```python
from build123d import *

# Parameters (mm, degrees)
SKETCH1_W           = 24
SKETCH1_H           = 34
SKETCH1_R           = 7.5
BOSS_EXTRUDE1_DEPTH = 28
SKETCH3_W           = 30
SKETCH3_H           = 12
BOSS_EXTRUDE2_DEPTH = 35.15
SKETCH4_R           = 11
CUT_EXTRUDE2_DEPTH  = 8
FILLET1_R           = 2
SKETCH5_W           = 12
SKETCH5_H           = 30
BOSS_EXTRUDE3_DEPTH = 10
SKETCH6_W           = 8
SKETCH6_H           = 5
CUT_EXTRUDE3_DEPTH  = 74.076141797
CUT_EXTRUDE4_REACH  = 87.286
SKETCH7_R           = 1
SKETCH8_R           = 4
CUT_EXTRUDE5_DEPTH  = 20
SKETCH9_R           = 7
CUT_EXTRUDE6_DEPTH  = 10


with BuildPart() as part:
    # Sketch1 → Boss-Extrude1 (new, symmetric)
    with BuildSketch(Plane.XY):
        with Locations((0, -5)):
            Rectangle(SKETCH1_W, SKETCH1_H)
        Circle(SKETCH1_R, mode=Mode.SUBTRACT)
    extrude(amount=BOSS_EXTRUDE1_DEPTH, both=True)

    # Sketch3 → Boss-Extrude2 (add)
    with BuildSketch(Plane.XZ.offset(22)):
        with Locations((0, 7.5)):
            Rectangle(SKETCH3_W, SKETCH3_H)
    extrude(amount=BOSS_EXTRUDE2_DEPTH)

    # Sketch4 → Cut-Extrude2 (cut)
    with BuildSketch(Plane.XY.offset(13.5)):
        with Locations((0, -43.15)):
            Circle(SKETCH4_R)
    extrude(amount=-CUT_EXTRUDE2_DEPTH, mode=Mode.SUBTRACT)

    # Fillet1
    fillet1_edges = [part.edges().sort_by_distance(p)[0] for p in [
        (0, -22, 1.5),
        (0, -22, 13.5),
    ]]
    fillet(fillet1_edges, radius=FILLET1_R)

    # Sketch5 → Boss-Extrude3 (add)
    with BuildSketch(Plane(origin=(0, 12, 0), x_dir=(1, 0, 0), z_dir=(0, 1, 0))):
        with Locations((6, 0)):
            Rectangle(SKETCH5_W, SKETCH5_H)
    extrude(amount=BOSS_EXTRUDE3_DEPTH)

    # Sketch6 → Cut-Extrude3 (cut, through all)
    with BuildSketch(Plane.XY.offset(15)):
        with Locations((4, 14.5)):
            Rectangle(SKETCH6_W, SKETCH6_H)
    extrude(amount=-CUT_EXTRUDE3_DEPTH, mode=Mode.SUBTRACT)

    # Sketch7 → Cut-Extrude4 (cut, up to next)
    with BuildSketch(Plane(origin=(0, 22, 0), x_dir=(1, 0, 0), z_dir=(0, 1, 0)), mode=Mode.PRIVATE) as cut_extrude4_sk1:
        with Locations(Location((4, 11, 0), (0, 0, 270))):
            Circle(SKETCH7_R)
    cut_extrude4_tool1 = extrude(cut_extrude4_sk1.sketch, amount=-CUT_EXTRUDE4_REACH, mode=Mode.PRIVATE) & part.part
    # Sketch7 → Cut-Extrude4 (cut, up to next)
    with BuildSketch(Plane(origin=(0, 22, 0), x_dir=(1, 0, 0), z_dir=(0, 1, 0)), mode=Mode.PRIVATE) as cut_extrude4_sk2:
        with Locations(Location((4, -11, 0), (0, 0, 270))):
            Circle(SKETCH7_R)
    cut_extrude4_tool2 = extrude(cut_extrude4_sk2.sketch, amount=-CUT_EXTRUDE4_REACH, mode=Mode.PRIVATE) & part.part
    add(cut_extrude4_tool1.solids().sort_by_distance((4, 22, -11))[0], mode=Mode.SUBTRACT)
    add(cut_extrude4_tool2.solids().sort_by_distance((4, 22, 11))[0], mode=Mode.SUBTRACT)

    # Sketch8 → Cut-Extrude5 (cut)
    with BuildSketch(Plane(origin=(12, 0, 0), x_dir=(0, 0, -1), z_dir=(1, 0, 0))):
        with Locations(Location((-14, -14, 0), (0, 0, 90))):
            Circle(SKETCH8_R)
        with Locations(Location((14, -14, 0), (0, 0, 90))):
            Circle(SKETCH8_R)
    extrude(amount=-CUT_EXTRUDE5_DEPTH, mode=Mode.SUBTRACT)

    # Sketch9 → Cut-Extrude6 (cut)
    with BuildSketch(Plane.XY.offset(5.5)):
        with Locations((0, -43.15)):
            Circle(SKETCH9_R)
    extrude(amount=-CUT_EXTRUDE6_DEPTH, mode=Mode.SUBTRACT)


solid = part.part
```
Geometry check sheet. Reference: the model listing, model coordinates, mm. A direction names the side the tool comes from. Coordinates: 2 decimals unless noted, no trailing zeros. Order: outer loops, then holes, each group sorted by start corner. A loop starts at its lowest first (then second) coordinate and runs counter-clockwise, first axis right, second up.
Item 1: Section check D-D (y = -40.5). Enter the section's corners in (x, z), plus the area to 3 significant figures.
Item 2: Section check B-B (z = -14). Enter the section's corners in (x, y), plus the area to 3 significant figures.
Item 3: Section check C-C (z = 11). Enter the section's corners in (x, y).
Item 4: Scan lines: line 1 along Z through (x, y) = (0.25, -14); line 2 along Y through (x, z) = (-4.75, -12); line 3 along X through (y, z) = (20.55, -11). Record each from-to range of solid material in increasing order.
Item 5: Depth check by flat-ended pin: pin 1 (8 mm diameter, centred on y = 13, z = -13, fed in from -X); pin 2 (23 mm diameter, centred on y = 7.5, z = -4, fed in from +X); pin 3 (1.5 mm diameter, centred on x = -6, z = 10.5, fed in from +Y); pin 4 (2.5 mm diameter, centred on x = 4, z = 11, fed in from +Y). Enter the tip coordinate at first touch or a pass-through.
Item 6: Tool access check on faces 4 (the flat face through (8, 14, 0)), 5 (the cylindrical face through (5.076, -52.909, 9.556)), 6 (the flat face through (0, -22, 22)), 7 (the flat face through (-8, -14, -14)). Record the directions out of +Z, -Z, +X, -X, +Y, -Y that give a thin tool (end or side, any length) a straight path to the whole face; none if there is none.
Item 7: Mould release check, pull along Y, two halves, no side actions. Record for faces 1 (the flat face through (-0.2, -50.3, 5.5)), 2 (the flat face through (-14, -22, 8)), 3 (the cylindrical face through (4.676, 19.535, -11.737)): released by +Y, released by -Y, zero draft, split by the parting line, or undercut.
Item 8: Section check A-A (y = 0). Enter the section's corners in (x, z).
Check sheet entries:
1. outline: (-15, 1.5) - (-6.48, 1.5) - (-6.48, 5.5) - (-10.68, 5.5) - (-10.68, 13.5) - (-15, 13.5) - close; (6.48, 1.5) - (15, 1.5) - (15, 13.5) - (10.68, 13.5) - (10.68, 5.5) - (6.48, 5.5) - close
1. area: 137 mm2
2. outline: (-12, -22) - (12, -22) - (12, -18) - (-8, -18) - (-8, -10) - (12, -10) - (12, 22) - (0, 22) - (0, 17) - (8, 17) - (8, 12) - (-12, 12) - close; hole circle Ø15 at (0, 0)
2. area: 559 mm2
3. outline: (-15, -57.15) - (15, -57.15) - (15, -22) - (12, -22) - (12, -16.65) - (-8, -16.65) - (-8, -11.35) - (12, -11.35) - (12, 22) - (5, 22) - (5, 17) - (8, 17) - (8, 12) - (-12, 12) - (-12, -22) - (-15, -22) - close; (0, 17) - (3, 17) - (3, 22) - (0, 22) - close; hole circle Ø22 at (0, -43.15); hole circle Ø15 at (0, 0)
4. line 1: z = -28 to -18, -10 to 10, 18 to 28
4. line 2: y = -22 to -17.46, -10.54 to -5.8, 5.8 to 12
4. line 3: x = 0 to 3, 5 to 12
5. pin 1: stops at x = -12
5. pin 2: stops at x = 12
5. pin 3: stops at y = 12
5. pin 4: stops at y = 22
6. face 4: +Z, -Z, -X
6. face 5: +Z
6. face 6: +Z, +X, -X, -Y
6. face 7: +X
7. face 1: undercut
7. face 2: released by +Y
7. face 3: zero draft
8. outline: (-12, -28) - (-7.5, -28) - (-7.5, 28) - (-12, 28) - close; (7.5, -28) - (12, -28) - (12, 28) - (7.5, 28) - close
